Check sheet for the modelled part. Datum: model origin and axes. Units: mm. A direction names the side the tool comes from. Round coordinates to 2 decimals unless told otherwise and drop trailing zeros. Order: outer loops, then holes, each group sorted by start corner. A loop starts at its lowest first (then second) coordinate and runs counter-clockwise, first axis right, second up.
```python
from build123d import *

# Parameters (mm, degrees)
SKETCH1_W           = 3.4
SKETCH1_H           = 8.7
SKETCH1_W_2         = 6
SKETCH1_H_2         = 42
BOSS_EXTRUDE1_DEPTH = 4
BOSS_EXTRUDE2_DEPTH = 4


with BuildPart() as part:
    # Sketch1 → Boss-Extrude1 (new body)
    with BuildSketch(Plane.XY):
        Polygon((-66.7, 30), (-66.7, -30), (55.3, -30), (60.740194605, -30), (60.740194605, -21), (58.8, -21), (51.3, -21), (51.3, 21), (58.8, 21), (60.740194605, 21), (60.740194605, 30), (55.3, 30), align=None)
        with Locations((-35.6, 20.65)):
            Rectangle(SKETCH1_W, SKETCH1_H, mode=Mode.SUBTRACT)
        with Locations((24.2, 20.65)):
            Rectangle(SKETCH1_W, SKETCH1_H, mode=Mode.SUBTRACT)
        with Locations((24.2, -20.65)):
            Rectangle(SKETCH1_W, SKETCH1_H, mode=Mode.SUBTRACT)
        with Locations((-24.2, 20.65)):
            Rectangle(SKETCH1_W, SKETCH1_H, mode=Mode.SUBTRACT)
        with Locations((-24.2, -20.65)):
            Rectangle(SKETCH1_W, SKETCH1_H, mode=Mode.SUBTRACT)
        with Locations((48.6, 20.65)):
            Rectangle(SKETCH1_W, SKETCH1_H, mode=Mode.SUBTRACT)
        with Locations((48.6, -20.65)):
            Rectangle(SKETCH1_W, SKETCH1_H, mode=Mode.SUBTRACT)
        with Locations((-35.6, -20.65)):
            Rectangle(SKETCH1_W, SKETCH1_H, mode=Mode.SUBTRACT)
        with Locations((-60, 20.65)):
            Rectangle(SKETCH1_W, SKETCH1_H, mode=Mode.SUBTRACT)
        with Locations((-60, -20.65)):
            Rectangle(SKETCH1_W, SKETCH1_H, mode=Mode.SUBTRACT)
        with Locations((-29.9, 0)):
            Rectangle(SKETCH1_W_2, SKETCH1_H_2, mode=Mode.SUBTRACT)
    extrude(amount=BOSS_EXTRUDE1_DEPTH)

    # Sketch2 → Boss-Extrude2 (add)
    with BuildSketch(Plane.XY):
        Polygon((-66.7, 30), (-66.7, 55), (-51.7, 55), (-37.557864376, 40.857864376), (31.598058981, 40.857864376), (45.740194605, 55), (60.740194605, 55), (60.740194605, 30), align=None)
    extrude(amount=BOSS_EXTRUDE2_DEPTH)


solid = part.part
```
Item 1: Sectioned sample at A-A (y = 14). Record the cut outline in (x, z), and give its area (3 significant figures).
Answer:
outline: (-66.7, 0) - (-32.9, 0) - (-32.9, 4) - (-66.7, 4) - close; (-26.9, 0) - (51.3, 0) - (51.3, 4) - (-26.9, 4) - close
area: 448 mm2
Item 2: Sectioned sample at D-D (x = 11). Record the cut outline in (y, z), and give its area (3 significant figures).
Answer:
outline: (-30, 0) - (40.86, 0) - (40.86, 4) - (-30, 4) - close
area: 283 mm2
Item 3: Release check for a two-part mould opening along X. For faces 1 (the flat face through (24, 25, 2)), 2 (the flat face through (56, 21, 2)) record: released by +X, released by -X, zero draft, split by the parting line, or undercut.
Answer:
face 1: undercut
face 2: zero draft
Item 4: Sectioned sample at B-B (x = -36). Record the cut outline in (y, z), and give its area (3 significant figures).
Answer:
outline: (-30, 0) - (-25, 0) - (-25, 4) - (-30, 4) - close; (-16.3, 0) - (16.3, 0) - (16.3, 4) - (-16.3, 4) - close; (25, 0) - (40.86, 0) - (40.86, 4) - (25, 4) - close
area: 214 mm2
Item 5: Access from +Z, -Z, +X, -X, +Y, -Y to the whole of each face (thin tool, end or side, straight path). Record for faces 3 (the flat face through (50.3, -21, 2)), 4 (the flat face through (38.57, 47.83, 1.97)), 5 (the flat face through (56, -21, 2)).
Answer:
face 3: +Z, -Z
face 4: +Z, -Z, +Y
face 5: +Z, -Z, +X
Item 6: Sectioned sample at C-C (z = 1.25). State how many separate pieces and enclosed holes the cut face has, and give its area (3 significant figures).
Answer:
separate pieces: 1
enclosed holes: 11
area: 8,710 mm2
Item 7: Go/stop test with flat-tipped pins: P1, Ø2, axis at x = -35, z = 1, coming from the +Y side; P2, Ø1, axis at y = -5, z = 0.5, coming from the +X side. Record where each tip stops, or that it passes through.
Answer:
P1: stops at y = 40.86
P2: stops at x = 51.3
Item 8: Scan lines: line 1 along X through (y, z) = (23.5, 2.55); line 2 along X through (y, z) = (7, 2.55); line 3 along Y through (x, z) = (23, 0.5). Record each from-to range of solid material in increasing order.
Answer:
line 1: x = -66.7 to -61.7, -58.3 to -37.3, -33.9 to -25.9, -22.5 to 22.5, 25.9 to 46.9, 50.3 to 60.74
line 2: x = -66.7 to -32.9, -26.9 to 51.3
line 3: y = -30 to -25, -16.3 to 16.3, 25 to 40.86
